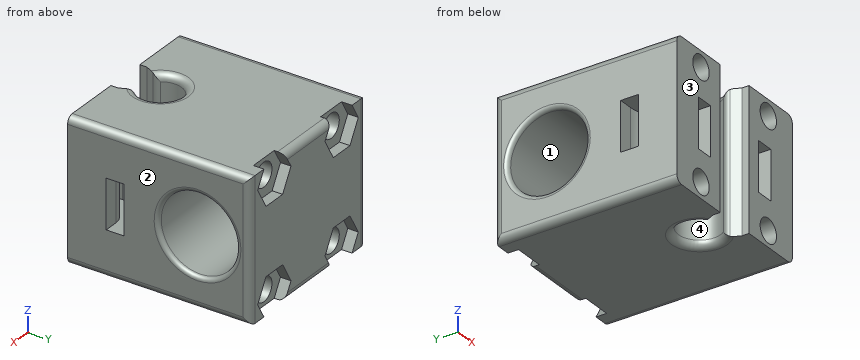
from build123d import *

# Parameters (mm, degrees)
CROQUIS1_W              = 24
CROQUIS1_H              = 19.999999388
SALIENTE_EXTRUIR1_DEPTH = 25
CORTAR_EXTRUIR1_DEPTH   = 60.75663166
CROQUIS4_R              = 1.7
CORTAR_EXTRUIR3_DEPTH   = 62.337415173
CROQUIS8_W              = 7
CROQUIS8_H              = 2.5
CORTAR_EXTRUIR7_DEPTH   = 1.5
CROQUIS3_R              = 5.575
CORTAR_EXTRUIR8_DEPTH   = 40
SALIENTE_EXTRUIR2_START = 1
CROQUIS13_W             = 9
CROQUIS13_H             = 19.999999388
CROQUIS13_R             = 1.7
CROQUIS13_W_2           = 2.5
CROQUIS13_H_2           = 7
SALIENTE_EXTRUIR2_DEPTH = 1
SALIENTE_EXTRUIR3_START = 1
CROQUIS14_W             = 9
CROQUIS14_H             = 19.999999388
CROQUIS14_R             = 1.7
CROQUIS14_W_2           = 2.5
CROQUIS14_H_2           = 7
SALIENTE_EXTRUIR3_DEPTH = 1
REDONDEO1_R             = 1
REDONDEO3_R             = 0.6


with BuildPart() as part:
    # Croquis1 → Saliente-Extruir1 (new body)
    with BuildSketch(Plane.XZ):
        with Locations((38.456466898, 14.319199476)):
            Rectangle(CROQUIS1_W, CROQUIS1_H)
    extrude(amount=-SALIENTE_EXTRUIR1_DEPTH)

    # Croquis2 → Cortar-Extruir1 (cut, through all)
    with BuildSketch(Plane.XY.offset(24.31919917)):
        with BuildLine():
            Line((35.456466898, 0), (36.335146555, 1.878679656))
            ThreePointArc((36.335146555, 1.878679656), (38.456466898, 7), (40.577787242, 1.878679656))
            Line((40.577787242, 1.878679656), (41.456466898, 0))
            Line((41.456466898, 0), (35.456466898, 0))
        make_face()
    extrude(amount=-CORTAR_EXTRUIR1_DEPTH, mode=Mode.SUBTRACT)

    # Croquis4 → Cortar-Extruir3 (cut, through all)
    with BuildSketch(Plane.XZ):
        with Locations(Location((31.464341614, 22.069199782, 0), (0, 0, 270))):
            Circle(CROQUIS4_R)
        with Locations(Location((45.448592182, 22.069199782, 0), (0, 0, 90))):
            Circle(CROQUIS4_R)
        with Locations(Location((45.448592182, 6.569198558, 0), (0, 0, 270))):
            Circle(CROQUIS4_R)
        with Locations(Location((31.464341614, 6.569198558, 0), (0, 0, 90))):
            Circle(CROQUIS4_R)
    extrude(amount=-CORTAR_EXTRUIR3_DEPTH, mode=Mode.SUBTRACT)

    # Cortar-Barrer2: sweep along a path in Croquis9
    with BuildLine(Plane(origin=(0, 0, 10.819199782), x_dir=(-1, 0, 0), z_dir=(0, 0, -1))) as cortar_barrer2_path:
        Line((-50.456466898, 6.999998763), (-48.456466898, 6.999998763))
        ThreePointArc((-48.456466898, 6.999998763), (-44.920932992, 5.535532669), (-43.456466898, 1.999998763))
        Line((-43.456466898, 1.999998763), (-43.456466898, -1.237e-06))
    # Croquis8 → Cortar-Barrer2 (sweep, cut)
    with BuildSketch(Plane(origin=(50.456466898, 0, 0), x_dir=(0, 0, -1), z_dir=(1, 0, 0))):
        with Locations((-14.319199782, 5.749998763)):
            Rectangle(CROQUIS8_W, CROQUIS8_H)
    cortar_barrer2 = sweep(path=cortar_barrer2_path.line, mode=Mode.SUBTRACT)

    # Simetría1: Cortar-Barrer2 across plane
    add(cortar_barrer2.mirror(Plane(origin=(38.456466898, 0, 0), x_dir=(0, 0, 1), z_dir=(1, 0, 0))), mode=Mode.SUBTRACT)

    # Croquis11 → Cortar-Extruir7 (cut)
    with BuildSketch(Plane(origin=(0, 25, 0), x_dir=(1, 0, 0), z_dir=(0, 1, 0))):
        Polygon((47.18064299, -19.069199782), (43.716541375, -19.069199782), (41.984490567, -22.069199782), (43.716541375, -25.069199782), (47.18064299, -25.069199782), (48.912693797, -22.069199782), align=None)
        Polygon((34.928443229, -22.069199782), (33.196392422, -19.069199782), (29.732290807, -19.069199782), (28.000239999, -22.069199782), (29.732290807, -25.069199782), (33.196392422, -25.069199782), align=None)
        Polygon((34.928443229, -6.569198558), (33.196392422, -3.569198558), (29.732290807, -3.569198558), (28.000239999, -6.569198558), (29.732290807, -9.569198558), (33.196392422, -9.569198558), align=None)
        Polygon((47.18064299, -9.569198558), (48.912693797, -6.569198558), (47.18064299, -3.569198558), (43.716541375, -3.569198558), (41.984490567, -6.569198558), (43.716541375, -9.569198558), align=None)
    extrude(amount=-CORTAR_EXTRUIR7_DEPTH, mode=Mode.SUBTRACT)

    # Croquis3 → Cortar-Extruir8 (cut)
    with BuildSketch(Plane(origin=(50.456466898, 0, 0), x_dir=(0, 0, -1), z_dir=(1, 0, 0))):
        with Locations((-14.31919917, 17.49999856)):
            Circle(CROQUIS3_R)
    extrude(amount=-CORTAR_EXTRUIR8_DEPTH, mode=Mode.SUBTRACT)

    # Croquis13 → Saliente-Extruir2 (add)
    with BuildSketch(Plane.XZ.offset(SALIENTE_EXTRUIR2_START)):
        with Locations((45.956466898, 14.319199476)):
            Rectangle(CROQUIS13_W, CROQUIS13_H)
        with Locations(Location((45.448592182, 22.069199782, 0), (0, 0, 270))):
            Circle(CROQUIS13_R, mode=Mode.SUBTRACT)
        with Locations(Location((45.448592182, 6.569198558, 0), (0, 0, 270))):
            Circle(CROQUIS13_R, mode=Mode.SUBTRACT)
        with Locations((44.706466898, 14.319199782)):
            Rectangle(CROQUIS13_W_2, CROQUIS13_H_2, mode=Mode.SUBTRACT)
    extrude(amount=-SALIENTE_EXTRUIR2_DEPTH)

    # Croquis14 → Saliente-Extruir3 (add)
    with BuildSketch(Plane.XZ.offset(SALIENTE_EXTRUIR3_START)):
        with Locations((30.956466898, 14.319199476)):
            Rectangle(CROQUIS14_W, CROQUIS14_H)
        with Locations(Location((31.464341614, 22.069199782, 0), (0, 0, 270))):
            Circle(CROQUIS14_R, mode=Mode.SUBTRACT)
        with Locations(Location((31.464341614, 6.569198558, 0), (0, 0, 270))):
            Circle(CROQUIS14_R, mode=Mode.SUBTRACT)
        with Locations((32.206466898, 14.319199782)):
            Rectangle(CROQUIS14_W_2, CROQUIS14_H_2, mode=Mode.SUBTRACT)
    extrude(amount=-SALIENTE_EXTRUIR3_DEPTH)

    # Redondeo1
    redondeo1_edges = [part.edges().sort_by_distance(p)[0] for p in [
        (38.456466898, 25, 24.31919917),
        (38.456466898, 25, 4.319199782),
        (26.456466898, 25, 14.319199476),
        (26.456466898, 12, 4.319199782),
        (26.456466898, 12, 24.31919917),
        (50.456466898, 12, 4.319199782),
        (50.456466898, 25, 14.319199476),
        (50.456466898, 12, 24.31919917),
        (40.577787242, 1.878679656, 14.319199476),
        (36.335146555, 1.878679656, 14.319199476),
        (38.456466898, 7, 4.319199782),
        (38.456466898, 7, 24.31919917),
    ]]
    fillet(redondeo1_edges, radius=REDONDEO1_R)

    # Redondeo3
    redondeo3_edges = [part.edges().sort_by_distance(p)[0] for p in [
        (26.456466898, 17.49999856, 19.89419917),
        (50.456466898, 17.49999856, 19.89419917),
    ]]
    fillet(redondeo3_edges, radius=REDONDEO3_R)


solid = part.part
Read the model definition and answer for the solid it produces. Units are mm, in the model's axes. Face numbers are marked on the shaded views. Give positions to 0.01 mm unless a question says otherwise; leave off trailing zeros. Answer as a JSON object with one key per item and string values. Group by question number.
1) Consider L1, parallel to Z at x = 34, y = 17.5; L2, parallel to X at y = 20.5, z = 21.75; L3, parallel to X at y = 4, z = 9. Determine where each line is inside the solid, lowest interval first. Write a range as from..to.
2) Find section A-A (y = 16.5). Count the separate pieces of the cut face and the enclosed holes in it, and give its area (3 significant figures).
3) Each of these flat-tipped pins is pushed along its axis until it touches: P1, Ø0.8, axis at x = 31.5, y = 24, coming from the -Z side; P2, Ø1.6, axis at x = 31, y = 24.5, coming from the +Z side; P3, Ø3.5, axis at x = 38.46, y = 4, coming from the -Z side; P4, Ø2.5, axis at x = 31, z = 20.5, coming from the +Y side. Where does it stop, or does it pass through?
4) The mould has two halves that part along Y. Classify the marked faces 1, 2, 3 and 4: +Y half, -Y half, draft (parallel to the pull), parting line (faces both ways), or undercut.
Values follow:
{
 "1": {"L1": "z = 4.32..8.74, 19.89..24.32", "L2": "x = 26.46..29.79, 33.13..43.78, 47.12..50.46", "L3": "x = 26.46..35.46, 41.46..50.46"},
 "2": {"separate pieces": "2", "enclosed holes": "4", "area": "179 mm2"},
 "3": {"P1": "stops at z = 9.57", "P2": "stops at z = 19.07", "P3": "passes through", "P4": "stops at y = 23.5"},
 "4": {"face 1": "undercut", "face 2": "draft", "face 3": "-Y half", "face 4": "undercut"}
}
